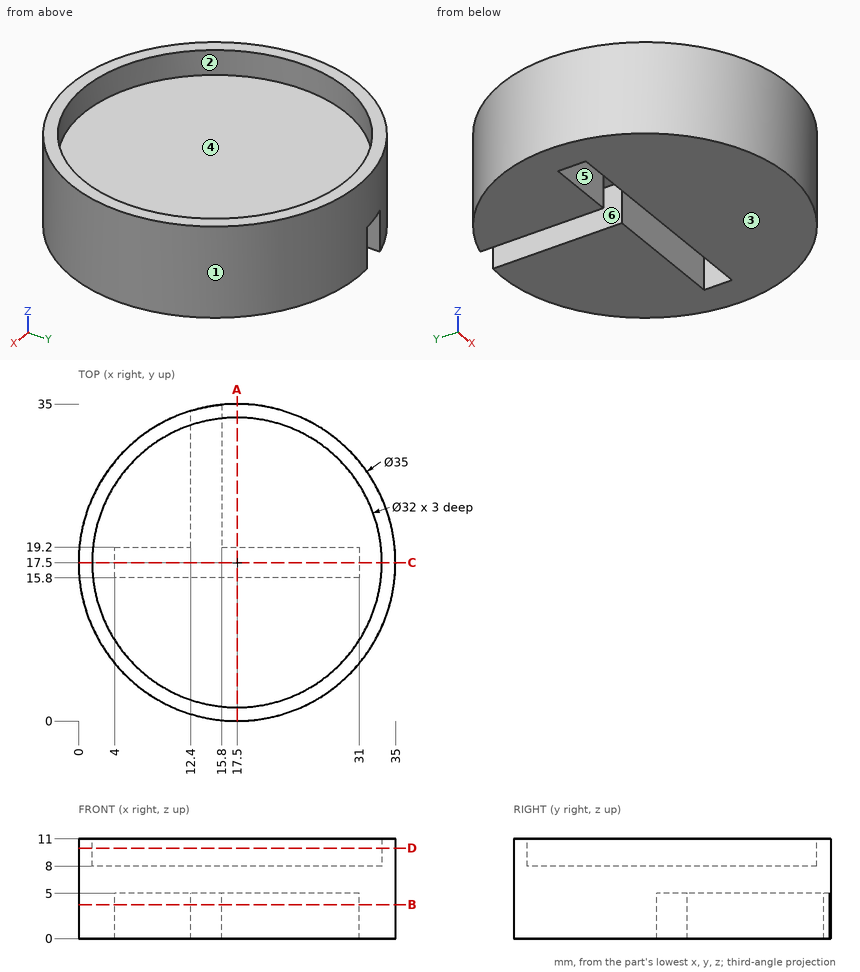
Check sheet for the drawn part. Datum: minimum x, y, z corner. Units: mm. A direction names the side the tool comes from. Coordinates: 2 decimals unless noted, no trailing zeros. Write each loop counter-clockwise with the first axis right and the second up, starting at its lowest first coordinate (ties: lowest second). Pieces come first, ordered by that corner, then holes. Notation, with made-up numbers: M 85,49.25 L 142,49.25 A23 cw 142,69.25 Z; hole C 58,-22 d1. An arc over 180 degrees is marked long. Use a Markdown table: item, result.
Q1. Draft check along X on the marked faces 1, 2 and 3. Enter one of: +X half, -X half, draft (parallel to the pull), parting line (faces both ways), or undercut.
Reply:
| item | result |
|---|---|
| face 1 | parting line |
| face 2 | undercut |
| face 3 | draft |
Q2. Go/stop test with flat-tipped pins: P1, Ø2.5, axis at y = 27.5, z = 1.5, coming from the +X side; P2, Ø16, axis at x = 18.5, y = 17.5, coming from the +Z side; P3, Ø1.5, axis at x = 25, z = 2.5, coming from the +Y side. Record where each tip stops, or that it passes through.
Reply:
| item | result |
|---|---|
| P1 | stops at x = 32.66 |
| P2 | stops at z = 8 |
| P3 | stops at y = 33.65 |
Q3. Thickness scan on line 1 (Y direction, x = 17.5, z = 9.9); line 2 (Z direction, x = 20, y = 6); line 3 (Y direction, x = 16.5, z = 2.25). Record the ranges inside material, lowest first.
Reply:
| item | result |
|---|---|
| line 1 | y = 0 to 1.5, 33.5 to 35 |
| line 2 | z = 0 to 8 |
| line 3 | y = 0.03 to 15.8, 19.2 to 34.97 |
Q4. Sectioned sample at D-D, the plane z = 10. Record the boundary of the cut face in (x, y).
Reply:
| item | result |
|---|---|
| outline | C 17.5,17.5 d35; hole C 17.5,17.5 d32 |
Q5. Sectioned sample at B-B, the plane z = 3.75. Record the boundary of the cut face in (x, y), plus the area to 3 significant figures.
Reply:
| item | result |
|---|---|
| outline | M 4,15.8 L 4,19.2 L 12.4,19.2 L 12.4,34.24 A17.5 ccw long 15.8,34.92 L 15.8,19.2 L 31,19.2 L 31,15.8 Z |
| area | 818 mm² |
Q6. Sectioned sample at C-C, the plane y = 17.5. Record the boundary of the cut face in (x, z).
Reply:
| item | result |
|---|---|
| outline | M 0,0 L 4,0 L 4,5 L 31,5 L 31,0 L 35,0 L 35,11 L 33.5,11 L 33.5,8 L 1.5,8 L 1.5,11 L 0,11 Z |
Q7. Sectioned sample at A-A, the plane x = 17.5. Record the boundary of the cut face in (y, z).
Reply:
| item | result |
|---|---|
| outline | M 0,0 L 15.8,0 L 15.8,5 L 19.2,5 L 19.2,0 L 35,0 L 35,11 L 33.5,11 L 33.5,8 L 1.5,8 L 1.5,11 L 0,11 Z |
Q8. Set-up check for the marked faces 4, 5 and 6: record each of +Z, -Z, +X, -X, +Y, -Y from which the full face is reachable in a straight line by a thin tool's end or side.
Reply:
| item | result |
|---|---|
| face 4 | +Z |
| face 5 | -Z |
| face 6 | -Z, +Y |
